Part model, mm, in its own coordinate system. A direction names the side the tool comes from. Round coordinates to 2 decimals unless told otherwise and drop trailing zeros. Write each loop counter-clockwise with the first axis right and the second up, starting at its lowest first coordinate (ties: lowest second). Pieces come first, ordered by that corner, then holes. Notation, with made-up numbers: M 43.5,45 L 80.5,45 A6 ccw 80.5,51 Z; hole C 26,16.5 d9. An arc over 180 degrees is marked long. Use a Markdown table: item, result. Add a question column.
1) Which spindle directions (+Z, -Z, +X, -X, +Y, -Y) get a long thin tool onto all of the face, cutting with end or side? Do faces 1 (the face through (-23, 29, -1.588)), 2 (the face through (-43.645, 174.564, -20.76)). Say none if no direction does.
2) Slice it at C-C on y = 22. Write the cut outline in (x, z), plus the area to 3 significant figures.
3) Drop flat-ended pins along their axis: P1, Ø6, axis at y = 83, z = -12.5, coming from the +X side; P2, Ø5.5, axis at y = 171.75, z = -22.22, coming from the -X side; P3, Ø1.3, axis at x = -26, z = -43.5, coming from the -Y side (3 decimals). Give the stop position or say it passes through.
4) Two-plate mould, pull along Z, no slides. Class faces 3 (the face through (-0.78, -143.5, -25.32)), 4 (the face through (-22, 37, 0)), 5 (the face through (-23, 37, -44.45)): released by +Z, released by -Z, zero draft, split by the parting line, or undercut.
5) Slice it at B-B on z = -4.5. Write the cut outline in (x, y), plus the area to 3 significant figures.
6) Wall check: probe 1 along X at (y, z) = (-59, -39). Give the ranges that are in metal, low to high.
7) Slice it at D-D on z = -28.5. Write the cut outline in (x, y), plus the area to 3 significant figures.
Autodesk Inventor part; units mm, degrees
ref_plane "YZ Plane" through (0, 0, 0) normal (1, 0, 0) x (0, 1, 0)
ref_plane "XZ Plane" through (0, 0, 0) normal (0, 1, 0) x (-1, 0, 0)
ref_plane "XY Plane" through (0, 0, 0) normal (0, 0, 1) x (1, 0, 0)
sketch "Sketch1" plane through (0, 0, 0) normal (0, 1, 0) x (-1, 0, 0)
  line L0 (0, 0) -> (44.45, 0)
  line L1 (44.45, 0) -> (44.45, -44.45)
  line L2 (44.45, -44.45) -> (0, -44.45)
  line L3 (0, -44.45) -> (0, 0)
  line L4 (42.8625, -1.5875) -> (1.5875, -1.5875)
  line L5 (1.5875, -1.5875) -> (1.5875, -42.8625)
  line L6 (1.5875, -42.8625) -> (42.8625, -42.8625)
  line L7 (42.8625, -42.8625) -> (42.8625, -1.5875)
  dimension "d0" = 44.45
  dimension "d2" = 1.5875
extrude "Extrusion1" add sketch "Sketch1" along normal mid plane 356.1949
ref_plane "Work Plane1" through (-22.225, -178.0974, -44.45) normal (1, 0, 0) x (0, 0, -1)
sketch "Sketch2" plane through (-44.45, -178.0974, 0) normal (-1, 0, 0) x (0, 0, 1)
  line L0 (-44.45, 356.1949) -> (0, 356.1949)
  line L1 (0, 356.1949) -> (0, 0)
  line L2 (-44.45, 356.1949) -> (-44.45, 0)
  point P0 (0, 178.0974)
  point P1 (-22.225, 349.8449)
  dimension "d5" = 6.35
  dimension "d17" = 22.225
hole "Hole1" at (-44.45, 171.7474, -22.225) direction (1, 0, 0) diameter 6.35 end through all
ref_plane "Work Plane2" through (-44.45, 178.0974, -22.225) normal (0, 0, 1) x (1, 0, 0)
sketch "Sketch3" plane through (-44.45, 178.0974, 0) normal (0, 0, 1) x (1, 0, 0)
  line L0 (44.45, -356.1949) -> (44.45, 0)
  line L1 (0, 0) -> (44.45, 0)
  line L2 (0, 0) -> (0, -356.1949)
  line L3 (44.45, -356.1949) -> (0, -356.1949)
  line L4 (1.5875, 0) -> (1.5875, -356.1949)
  line L5 (42.8625, -356.1949) -> (42.8625, 0)
  line L6 (1.5875, -356.1949) -> (42.8625, -356.1949)
  line L7 (1.5875, -356.1949) -> (42.8625, -356.1949)
  line L8 (42.8625, -356.1949) -> (42.8625, -294.2824)
  line L9 (42.8625, -294.2824) -> (1.5875, -294.2824)
  line L10 (1.5875, -294.2824) -> (1.5875, -356.1949)
  point P0 (44.45, -178.0974)
  dimension "d14" = 61.9125
extrude "Extrusion2" cut sketch "Sketch3" against normal through all contours L3 L4 L9 L5
sketch "Sketch4" plane through (-44.45, -178.0974, 0) normal (-1, 0, 0) x (0, 0, 1)
  line L0 (-44.45, 356.1949) -> (-44.45, 0)
  line L1 (0, 0) -> (-44.45, 0)
  point P0 (0, 178.0974)
  point P1 (-22.225, 20.6502)
  dimension "d18" = 22.225
  dimension "d19" = 20.6502
hole "Hole2" at (-44.45, -157.4472, -22.225) direction (1, 0, 0) diameter 28.575 end through all
properties part number "CAR_025_KickerBar" material "Aluminum 6061"
Entries:
| question | item | result |
|---|---|---|
| 1 | face 1 | +Y, -Y |
| 1 | face 2 | +X, -X |
| 2 | outline | M -44.45,-44.45 L 0,-44.45 L 0,0 L -44.45,0 Z; hole M -42.86,-42.86 L -1.59,-42.86 L -1.59,-1.59 L -42.86,-1.59 Z |
| 2 | area | 272 mm^2 |
| 3 | P1 | stops at x = 0 |
| 3 | P2 | passes through |
| 3 | P3 | stops at y = -116.185 |
| 4 | face 3 | undercut |
| 4 | face 4 | released by +Z |
| 4 | face 5 | released by -Z |
| 5 | outline | M -44.45,-178.1 L -42.86,-178.1 L -42.86,178.1 L -44.45,178.1 Z; M -1.59,-178.1 L 0,-178.1 L 0,178.1 L -1.59,178.1 Z |
| 5 | area | 1,130 mm^2 |
| 6 | probe 1 | x = -44.45 to -42.86, -1.59 to 0 |
| 7 | outline | M -44.45,-178.1 L -42.86,-178.1 L -42.86,-170.28 L -44.45,-170.28 Z; M -44.45,-144.61 L -42.86,-144.61 L -42.86,178.1 L -44.45,178.1 Z; M -1.59,-178.1 L 0,-178.1 L 0,-170.28 L -1.59,-170.28 Z; M -1.59,-144.61 L 0,-144.61 L 0,178.1 L -1.59,178.1 Z |
| 7 | area | 1,050 mm^2 |
